Build history of the part. All positions in model axes, mm. A direction names the side the tool comes from. Give positions to 0.01 mm unless a question says otherwise; leave off trailing zeros. Order: outer loops, then holes, each group sorted by start corner. A loop starts at its lowest first (then second) coordinate and runs counter-clockwise, first axis right, second up. Notation, with made-up numbers: M 14.5,54 L 51.5,54 A15 cw 51.5,63 Z; hole C -5.5,86.5 d8. An arc over 180 degrees is marked long. One line per item, written item: value.
Autodesk Inventor part; units mm, degrees
ref_plane "YZ Plane" through (0, 0, 0) normal (1, 0, 0) x (0, 1, 0)
ref_plane "XZ Plane" through (0, 0, 0) normal (0, 1, 0) x (-1, 0, 0)
ref_plane "XY Plane" through (0, 0, 0) normal (0, 0, 1) x (1, 0, 0)
sketch "Sketch1" plane through (0, 0, 0) normal (0, 0, 1) x (1, 0, 0)
  line L0 (-24, 48) -> (-24, 51)
  line L1 (-24, 51) -> (-40, 51)
  line L2 (-40, 51) -> (-40, 48)
  line L3 (0, 32) -> (3, 32)
  line L4 (3, 32) -> (3, 16)
  line L5 (3, 16) -> (0, 16)
  line L6 (-40, 0) -> (-40, -3)
  line L7 (-40, -3) -> (-24, -3)
  line L8 (-24, -3) -> (-24, 0)
  line L9 (-64, 16) -> (-67, 16)
  line L10 (-67, 16) -> (-67, 32)
  line L11 (-67, 32) -> (-64, 32)
  line L12 (-64, 48) -> (-40, 48)
  line L13 (-24, 48) -> (0, 48)
  line L14 (-64, 0) -> (-64, 16)
  line L15 (-64, 32) -> (-64, 48)
  line L16 (0, 0) -> (-24, 0)
  line L17 (-40, 0) -> (-64, 0)
  line L18 (0, 48) -> (0, 32)
  line L19 (0, 16) -> (0, 0)
  point P0 (0, 0)
  dimension "d3" = 16
  dimension "d4" = 16
  dimension "d8" = 64
  dimension "d9" = 48
  dimension "d10" = 3
  dimension "d11" = 3
  dimension "d12" = 24
  dimension "d13" = 24
  dimension "d14" = 16
  dimension "d15" = 3
extrude "Plate1" add sketch "Sketch1" along normal blind 3
sketch "Sketch2" plane through (0, 0, 3) normal (0, 0, 1) x (1, 0, 0)
  circle A0 centre (-32, 24) radius 10
  line L0 (-67, 32) -> (-67, 16)
  line L1 (-40, 51) -> (-24, 51)
  line L2 (0, 0) -> (0, 16)
  circle A1 centre (-32, 24) radius 16.5
  circle A2 centre (-32, 24) radius 20
  line L3 (0, 0) -> (-24, 0)
  line L4 (-64, 32) -> (-64, 48)
  line L5 (0, 48) -> (0, 32)
  line L6 (-64, 48) -> (-40, 48)
  line L7 (-64, 0) -> (-40, 0)
  line L8 (-52, 24) -> (-12, 24)
  line L9 (-32, 44) -> (-32, 4)
  line L10 (-17.8579, 38.1421) -> (-46.1421, 9.8579)
  line L11 (-17.8579, 9.8579) -> (-46.1421, 38.1421)
  line L12 (-22.6485, 37.5941) -> (-20.1392, 40.1035)
  line L13 (-18.4059, 14.6485) -> (-15.8965, 12.1392)
  line L14 (-41.3515, 10.4059) -> (-43.8608, 7.8965)
  line L15 (-45.5941, 33.3515) -> (-48.1035, 35.8608)
  circle A3 centre (-32, 24) radius 13
  circle A4 centre (-54, 5) radius 2.5
  circle A5 centre (-54, 13) radius 2.5
  line L16 (-64, 0) -> (-64, 16)
  point P0 (-32, 24)
  point P1 (-17.1512, 13.3939)
  point P2 (-32, 37)
  point P3 (-22.8076, 33.1924)
  point P4 (-32, 40.5)
  point P5 (-19, 24)
  point P6 (-22.8076, 14.8076)
  point P7 (-48.5, 24)
  point P8 (-32, 11)
  point P9 (-41.1924, 14.8076)
  point P10 (-32, 7.5)
  point P11 (-15.5, 24)
  point P12 (-45, 24)
  point P13 (-41.1924, 33.1924)
  point P14 (-43.6673, 35.6673)
  point P15 (-32, 24)
  point P16 (-20.3327, 12.3327)
  dimension "d17" = 20
  dimension "d21" = 3.5
  dimension "d24" = 24
  dimension "d25" = 32
  dimension "d26" = 45
  dimension "d27" = 3
  dimension "d28" = 3
  dimension "d29" = 3
  dimension "d30" = 3
  dimension "d31" = 3
  dimension "d34" = 5
  dimension "d35" = 5
  dimension "d36" = 5
  dimension "d37" = 10
  dimension "d38" = 8
  dimension "d39" = 3.5
extrude "Extrusion1" cut sketch "Sketch2" against normal through all contours L8 L10 A0 | A0 L11 L8 | L10 L9 A0 | A0 L9 L11 | L8 A1 L11 A3 | L10 A0 L8 | L11 A0 L9 | L9 A0 L10 | L8 A0 L11 | A3 L9 A1 L10 | A1 L12 A2 L10 | L9 A1 L10 A3 | A1 L13 A2 L11 | L8 A1 L11 A3 | A1 L14 A2 L10 | A1 L15 A2 L11 | A4 | A5
equation "\"d16\" = Thickness"
equation "\"BendRadius\" = Thickness"
equation "\"BendReliefWidth\" = Thickness"
equation "\"BendReliefDepth\" = 0.5 * Thickness"
equation "\"CornerReliefSize\" = 4 * Thickness"
equation "\"MinimumRemnant\" = 2 * Thickness"
equation "\"TransitionRadius\" = BendRadius"
equation "\"JacobiRadiusSize\" = BendRadius"
equation "\"GapSize\" = Thickness"
properties part number "back plate" material "Hardboard"
1) Saw through at C-C, the plane x = -29.5. Write the cut outline in (y, z), then the cut area to 3 significant figures.
Check values:
outline: M -3,0 L 14.32,0 L 14.32,3 L -3,3 Z; M 33.68,0 L 36.76,0 L 36.76,3 L 33.68,3 Z; M 40.31,0 L 51,0 L 51,3 L 40.31,3 Z
area: 93.2 mm^2
2) Mould opens along X. For faces 1 (the face through (-32, 12, 3)), 2 (the face through (-20, 36, 2)), 3 (the face through (-24, 49, 1)) say: released by +X, released by -X, zero draft, split by the parting line, or undercut.
Check values:
face 1: zero draft
face 2: undercut
face 3: released by +X
3) Tool access for faces 4 (the face through (1, 32, 1)), 5 (the face through (-27, 36, 2)), 6 (the face through (-52, 48, 1)): list every direction of +Z, -Z, +X, -X, +Y, -Y with a clear straight run to the whole face (end or side of a thin tool).
Check values:
face 4: +Z, -Z, +X, +Y
face 5: +Z, -Z
face 6: +Z, -Z, -X, +Y
4) Drill centre lines: probe 1 along Y at (x, z) = (-54, 2.25); probe 2 along Y at (x, z) = (-32.5, 1.8); probe 3 along X at (y, z) = (25, 0.65). Where is each one in solid material? Low to high. Write a range as from..to.
Check values:
probe 1: 0..2.5, 7.5..10.5, 15.5..48
probe 2: -3..7.51, 11.01..14.01, 33.99..51
probe 3: -67..-48.47, -44.96..-41.95, -22.05..3
5) Saw through at A-A, the plane y = 3.5. Write the cut outline in (x, z).
Check values:
outline: M -64,0 L -56,0 L -56,3 L -64,3 Z; M -52,0 L 0,0 L 0,3 L -52,3 Z
6) Saw through at D-D, the plane y = 26. Write the cut outline in (x, z).
Check values:
outline: M -67,0 L -48.38,0 L -48.38,3 L -67,3 Z; M -44.85,0 L -41.8,0 L -41.8,3 L -44.85,3 Z; M -22.2,0 L 3,0 L 3,3 L -22.2,3 Z
7) Saw through at B-B, the plane y = 13. Write the cut outline in (x, z), then the cut area to 3 significant figures.
Check values:
outline: M -64,0 L -56.5,0 L -56.5,3 L -64,3 Z; M -51.5,0 L -43,0 L -43,3 L -51.5,3 Z; M -38.93,0 L -21,0 L -21,3 L -38.93,3 Z; M -16.76,0 L 0,0 L 0,3 L -16.76,3 Z
area: 152 mm^2
8) Pin check, flat tips, straight feed: pin 1 (0.9 mm diameter, centred on y = 11, z = 2, fed in from -X); pin 2 (1 mm diameter, centred on x = -6.5, z = 2, fed in from +Y); pin 3 (0.9 mm diameter, centred on x = -16.5, z = 2, fed in from -Y). Stop position of each tip, or through.
Check values:
pin 1: x = -64
pin 2: y = 48
pin 3: y = 0
